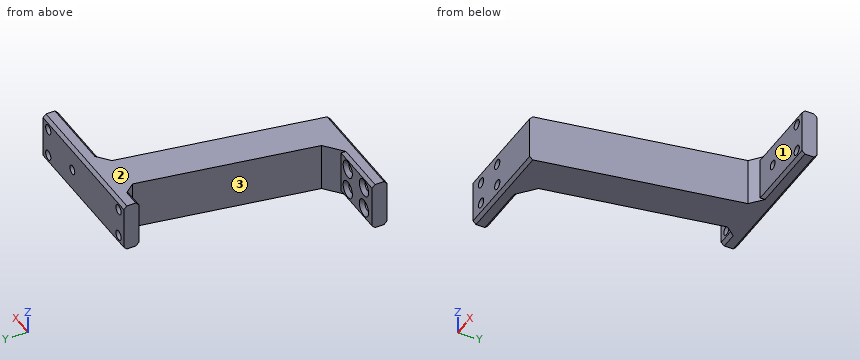
Autodesk Inventor part; units mm, degrees
ref_plane "YZ Plane" through (0, 0, 0) normal (1, 0, 0) x (0, 1, 0)
ref_plane "XZ Plane" through (0, 0, 0) normal (0, 1, 0) x (-1, 0, 0)
ref_plane "XY Plane" through (0, 0, 0) normal (0, 0, 1) x (1, 0, 0)
sketch "Sketch1" plane through (0, 0, 0) normal (0, 0, 1) x (1, 0, 0)
  line L0 (483.5261, -135.8063) -> (507.8593, 2.1937)
  line L1 (509.6225, 12.1937) -> (464.6225, 12.1937)
  line L2 (464.6225, 14.1937) -> (464.6225, 12.1937) construction
  line L3 (464.6225, 12.1937) -> (564.6225, 12.1937) construction
  line L4 (564.6225, 12.1937) -> (564.6225, 14.1937) construction
  line L5 (564.6225, 14.1937) -> (464.6225, 14.1937) construction
  line L6 (564.6225, 14.1937) -> (464.6225, 14.1937) construction
  line L7 (564.6225, 14.1937) -> (564.6225, 30.1937) construction
  line L8 (552.6225, 30.1937) -> (564.6225, 30.1937) construction
  arc A0 (536.6225, 30.1937) -> (552.6225, 30.1937) centre (544.6225, 30.1937) ccw construction
  line L9 (527.1225, 30.1937) -> (536.6225, 30.1937) construction
  arc A1 (502.1225, 30.1937) -> (527.1225, 30.1937) centre (514.6225, 30.1937) ccw construction
  line L10 (492.6225, 30.1937) -> (502.1225, 30.1937) construction
  arc A2 (476.6225, 30.1937) -> (492.6225, 30.1937) centre (484.6225, 30.1937) ccw construction
  line L11 (464.6225, 30.1937) -> (476.6225, 30.1937) construction
  line L12 (464.6225, 14.1937) -> (464.6225, 30.1937) construction
  line L13 (464.6225, 12.1937) -> (464.6225, 2.1937)
  line L14 (464.6225, 2.1937) -> (482.4736, 2.1937)
  line L15 (482.4736, 2.1937) -> (459.9038, -125.8063)
  line L16 (564.6225, 12.1937) -> (464.6225, 12.1937)
  line L17 (464.6225, 12.1937) -> (464.6225, 7.1937)
  line L18 (483.5261, -135.8063) -> (413.5261, -135.8063)
  line L19 (413.5261, -135.8063) -> (413.5261, -125.8063)
  line L20 (413.5261, -125.8063) -> (459.9038, -125.8063)
  line L21 (507.8593, 2.1937) -> (564.6225, 2.1937)
  line L22 (564.6225, 2.1937) -> (564.6225, 12.1937)
  point P0 (0, 0)
  dimension "d16" = 45
  dimension "d17" = 25
  dimension "d25" = 10
  dimension "d26" = 80
  dimension "d58" = 70
  dimension "d59" = 10
  dimension "d62" = 150
extrude "Extrusion1" add sketch "Sketch1" against normal blind 32
chamfer "Chamfer5" distance 5 angle 45 1 edges at (507.8593, 2.1937, -16)
chamfer "Chamfer8" distance 5 angle 45 1 edges at (482.4736, 2.1937, -16)
chamfer "Chamfer11" distance 8 angle 45 1 edges at (459.9038, -125.8063, -16)
chamfer "Chamfer6" distance 2 angle 45 10 edges at (448.5261, -135.8063, 0) (448.5261, -135.8063, -32) (514.6225, 12.1937, 0) (514.6225, 12.1937, -32) (538.7409, 2.1937, -32) (538.7409, 2.1937, 0) (471.0481, 2.1937, -32) (471.0481, 2.1937, 0) (432.715, -125.8063, -32) (432.715, -125.8063, 0)
sketch "Sketch9" plane through (464.6225, 12.1937, -2) normal (0, 1, 0) x (1, 0, 0)
  circle A0 centre (6.5, 23.5) radius 3.2
  circle A1 centre (6.5, 4.5) radius 3.2
  circle A2 centre (36.3, 14) radius 3
  circle A3 centre (63.7, 14) radius 3
  circle A4 centre (93.5, 23.5) radius 3.2
  circle A5 centre (93.5, 4.5) radius 3.2
  point P0 (-464.6225, -2)
extrude "Extrusion6" cut sketch "Sketch9" against normal blind 32 contours A0 | A1 | A3 | A4 | A5
sketch "Sketch10" plane through (413.5261, -135.8063, -30) normal (0, -1, 0) x (1, 0, 0)
  line L0 (70, 28) -> (70, 0)
  line L1 (0, 28) -> (0, 0)
  circle A0 centre (10, 21.5) radius 3.2
  circle A1 centre (10, 6.5) radius 3.2
  circle A2 centre (30, 21.5) radius 3.2
  circle A3 centre (30, 6.5) radius 3.2
  line L2 (10, 21.5) -> (30, 21.5) construction
  line L3 (30, 21.5) -> (30, 6.5) construction
  line L4 (30, 6.5) -> (10, 6.5) construction
  line L5 (10, 6.5) -> (10, 21.5) construction
  line L6 (70, 0) -> (0, 0)
  line L7 (0, 28) -> (70, 28)
  point P0 (-413.5261, 30)
  point P1 (10, 14)
  point P2 (0, 14)
  dimension "d51" = 6.4
  dimension "d52" = 10
  dimension "d53" = 20
  dimension "d54" = 15
extrude "Extrusion7" cut sketch "Sketch10" against normal blind 32 contours A0 | A1 | A2 | A3
chamfer "Chamfer10" distance 2.5 angle 45 4 edges at (440.3261, -125.8063, -23.5) (440.3261, -125.8063, -8.5) (420.3261, -125.8063, -23.5) (420.3261, -125.8063, -8.5)
properties part number "AXLG" material "PC/ABS Plastic"
Geometry: final body of the model. Coordinates: model frame, mm. Face numbers are marked on the shaded views. Round coordinates to 2 decimals unless told otherwise and drop trailing zeros. Loops run counter-clockwise (first coordinate to the right, second up) from the corner with the lowest first, then second, coordinate; pieces in that order, holes last.
Item 1: Line query: L1, parallel to X at y = 8, z = -6; L2, parallel to X at y = 9.5, z = -25.5; L3, parallel to X at y = 8, z = -16. Output: solid intervals per line, ascending.
Checked values:
L1: x = 464.62 to 467.96, 474.28 to 554.96, 561.28 to 564.62
L2: x = 464.62 to 467.92, 474.32 to 554.92, 561.32 to 564.62
L3: x = 464.62 to 525.32, 531.32 to 564.62
Item 2: Section A-A, the plane z = -16. Output: boundary loops of the cut face in (x, y), plus the area to 3 significant figures.
Checked values:
outline: (413.53, -135.81) - (483.53, -135.81) - (506.99, -2.73) - (512.86, 2.19) - (525.32, 2.19) - (525.32, 12.19) - (464.62, 12.19) - (464.62, 2.19) - (477.47, 2.19) - (481.61, -2.73) - (461.29, -117.93) - (451.9, -125.81) - (413.53, -125.81) - close; (531.32, 2.19) - (564.62, 2.19) - (564.62, 12.19) - (531.32, 12.19) - close
area: 4,950 mm2
Item 3: Section C-C, the plane y = -59. Output: boundary loops of the cut face in (x, z).
Checked values:
outline: (471.68, -32) - (497.07, -32) - (497.07, 0) - (471.68, 0) - close
Item 4: Mould query, pull axis Y, two halves, no side actions, for the marked faces 1, 2 and 3. Classes: released by +Y, released by -Y, zero draft, split by the parting line, or undercut.
Checked values:
face 1: released by -Y
face 2: zero draft
face 3: undercut
Item 5: Contact query for flat-ended pins moving along their axis: P1, Ø10, axis at x = 423.53, z = -8.5, coming from the +Y side; P2, Ø8.5, axis at x = 533, z = -18, coming from the -Y side; P3, Ø5, axis at x = 443.53, z = -23.5, coming from the -Y side; P4, Ø4, axis at y = -42.5, z = -19.5, coming from the -X side. Output: stop coordinate, or through.
Checked values:
P1: stops at y = -126.5
P2: stops at y = 2.19
P3: passes through
P4: stops at x = 474.24
Item 6: Section B-B, the plane y = -105. Output: boundary loops of the cut face in (x, z), plus the area to 3 significant figures.
Checked values:
outline: (463.57, -32) - (488.96, -32) - (488.96, 0) - (463.57, 0) - close
area: 812 mm2
